from build123d import *

# Parameters (mm, degrees)
SKETCH1_R           = 10.75
BOSS_EXTRUDE1_DEPTH = 40
SKETCH4_R           = 21
SKETCH4_R_2         = 2
BOSS_EXTRUDE3_DEPTH = 5
BOSS_EXTRUDE5_DEPTH = 4
SKETCH7_R           = 10.75
BOSS_EXTRUDE6_DEPTH = 40


with BuildPart() as part:
    # Sketch1 → Boss-Extrude1 (new body)
    with BuildSketch(Plane(origin=(0, 0, 0), x_dir=(0, 0, -1), z_dir=(1, 0, 0))):
        Circle(SKETCH1_R)
    extrude(amount=BOSS_EXTRUDE1_DEPTH)

    # Sketch4 → Boss-Extrude3 (add)
    with BuildSketch(Plane.ZY):
        Circle(SKETCH4_R)
        with Locations((-11, 11)):
            Circle(SKETCH4_R_2, mode=Mode.SUBTRACT)
        with Locations((11, 11)):
            Circle(SKETCH4_R_2, mode=Mode.SUBTRACT)
        with Locations((11, -11)):
            Circle(SKETCH4_R_2, mode=Mode.SUBTRACT)
        with Locations((-11, -11)):
            Circle(SKETCH4_R_2, mode=Mode.SUBTRACT)
    extrude(amount=BOSS_EXTRUDE3_DEPTH)

    # Sketch6 → Boss-Extrude5 (add)
    with BuildSketch(Plane(origin=(40, 0, 0), x_dir=(0, 0, -1), z_dir=(1, 0, 0))):
        with BuildLine():
            Line((-2.25, 6.511898021), (2.25, 6.511898021))
            Line((2.25, 6.511898021), (2.25, 10.511898021))
            ThreePointArc((2.25, 10.511898021), (0, -10.75), (-2.25, 10.511898021))
            Line((-2.25, 10.511898021), (-2.25, 6.511898021))
        make_face()
    extrude(amount=BOSS_EXTRUDE5_DEPTH)

    # Sketch7 → Boss-Extrude6 (add)
    with BuildSketch(Plane(origin=(44, 0, 0), x_dir=(0, 0, -1), z_dir=(1, 0, 0))):
        Circle(SKETCH7_R)
    extrude(amount=BOSS_EXTRUDE6_DEPTH)


solid = part.part
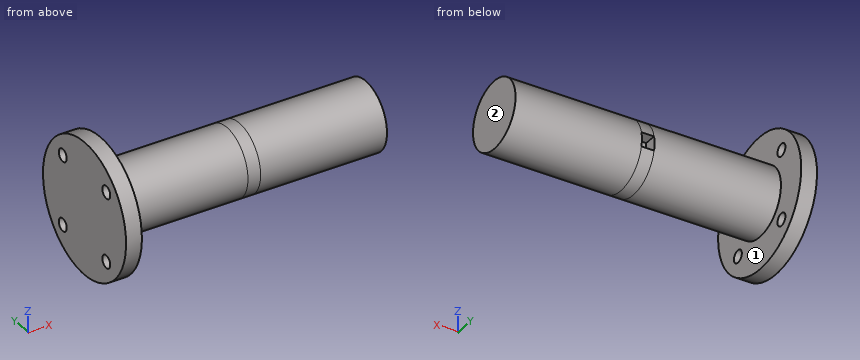
Model file for the job. Use its own axes, mm. Face numbers are marked on the shaded views. A direction names the side the tool comes from. Give positions to 0.01 mm unless a question says otherwise; leave off trailing zeros. Write each loop counter-clockwise with the first axis right and the second up, starting at its lowest first coordinate (ties: lowest second). Pieces come first, ordered by that corner, then holes. Notation, with made-up numbers: (-3.75, 80) -> (37.25, 80) arc R29 cw to (37.25, 110) -> close; hole circle Ø11 at (45, -12). An arc over 180 degrees is marked (long way). Write item = value, one per line.
(1) Tool access for the marked faces 1 and 2: list every direction of +Z, -Z, +X, -X, +Y, -Y with a clear straight run to the whole face (end or side of a thin tool).
Determined:
face_1 = +X
face_2 = +Z, -Z, +X, +Y, -Y
(2) Flat gauge pins, fed straight in: P1, Ø6, axis at x = 4.5, y = 14.5, coming from the -Z side; P2, Ø5, axis at y = 11, z = -11, coming from the -X side; P3, Ø4, axis at x = 29, z = -11, coming from the -Y side; P4, Ø2, axis at x = 41, y = 8, coming from the +Z side. Where does each tip first touch, or does it go through?
Determined:
P1 = through
P2 = -5
P3 = -5.88
P4 = 8.16
(3) Slice it at D-D, the plane z = 6. Give the cut face in (x, y), then the cut area to 3 significant figures.
Determined:
outline = (-5, -20.12) -> (0, -20.12) -> (0, -8.92) -> (84, -8.92) -> (84, 8.92) -> (0, 8.92) -> (0, 20.12) -> (-5, 20.12) -> close
area = 1,700 mm2
(4) Slice it at B-B, the plane z = 0. Give the cut face in (x, y), then the cut area to 3 significant figures.
Determined:
outline = (-5, -21) -> (0, -21) -> (0, -10.75) -> (84, -10.75) -> (84, 10.75) -> (44, 10.75) -> (44, 6.51) -> (40, 6.51) -> (40, 10.75) -> (0, 10.75) -> (0, 21) -> (-5, 21) -> close
area = 2,000 mm2
(5) Probe line 1 along Y through (x, z) = (-3, -11); line 2 along X through (y, z) = (-10, -13); line 3 along Z through (x, y) = (53.5, -0.5). List the from-to ranges inside material, lowest first.
Determined:
line_1 = -17.89 to -13, -9 to 9, 13 to 17.89
line_2 = -5 to 0
line_3 = -10.74 to 10.74
(6) Slice it at A-A, the plane y = 0. Give the cut face in (x, z), then the cut area to 3 significant figures.
Determined:
outline = (-5, -21) -> (0, -21) -> (0, -10.75) -> (84, -10.75) -> (84, 10.75) -> (0, 10.75) -> (0, 21) -> (-5, 21) -> close
area = 2,020 mm2
(7) Slice it at C-C, the plane x = 31. Give the cut face in (y, z).
Determined:
outline = circle Ø21.5 at (0, 0)
